Check sheet for the drawn part. Datum: minimum x, y, z corner. Units: mm. A direction names the side the tool comes from. Round coordinates to 2 decimals unless told otherwise and drop trailing zeros. Loops run counter-clockwise (first coordinate to the right, second up) from the corner with the lowest first, then second, coordinate; pieces in that order, holes last. Notation, with made-up numbers: (62.25, 68.5) - (83.25, 68.5) arc R22 cw to (83.25, 104.5) - close; hole circle Ø2 at (62.25, -40). An arc over 180 degrees is marked (long way). Use CSV: the item, a comma, the result in double quotes.
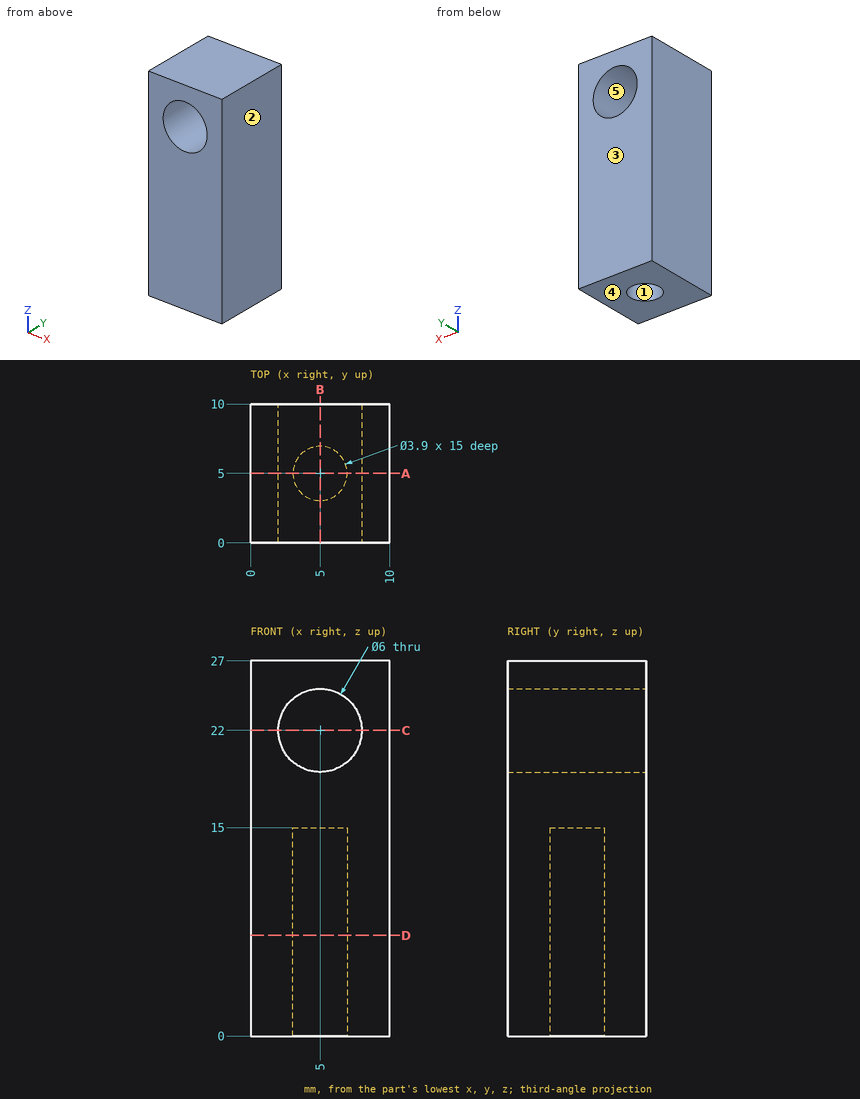
1) Gauge pin test, flat ends, axial feed: pin 1 Ø3 at (x, z) = (4, 22.5) entering from -Y; pin 2 Ø3.5 at (x, y) = (5, 5) entering from -Z. Record the tip position at first contact, or that the pin passes through.
Returned:
pin 1,"passes through"
pin 2,"stops at z = 15"
2) Access from +Z, -Z, +X, -X, +Y, -Y to the whole of each face (thin tool, end or side, straight path). Record for the marked faces 1 and 2.
Returned:
face 1,"-Z"
face 2,"+Z, -Z, +X, +Y, -Y"
3) Cross-section at C-C, the plane z = 22. Record the cut outline in (x, y), then the cut area to 3 significant figures.
Returned:
outline,"(0, 0) - (2, 0) - (2, 10) - (0, 10) - close; (8, 0) - (10, 0) - (10, 10) - (8, 10) - close"
area,"40.0 mm²"
4) Cross-section at B-B, the plane x = 5. Record the cut outline in (y, z).
Returned:
outline,"(0, 0) - (3.05, 0) - (3.05, 15) - (6.95, 15) - (6.95, 0) - (10, 0) - (10, 19) - (0, 19) - close; (0, 25) - (10, 25) - (10, 27) - (0, 27) - close"
5) Thickness scan on probe 1 along Y at (x, z) = (5, 10); probe 2 along Z at (x, y) = (5, 3.5). Record the ranges inside material, lowest first. Write a range as [from, to].
Returned:
probe 1,"y = [0, 3.05], [6.95, 10]"
probe 2,"z = [15, 19], [25, 27]"
6) Cross-section at A-A, the plane y = 5. Record the cut outline in (x, z), then the cut area to 3 significant figures.
Returned:
outline,"(0, 0) - (3.05, 0) - (3.05, 15) - (6.95, 15) - (6.95, 0) - (10, 0) - (10, 27) - (0, 27) - close; hole circle Ø6 at (5, 22)"
area,"183 mm²"
7) Mould release check, pull along Z, two halves, no side actions. Record for the marked faces 3, 4 and 5: +Z half, -Z half, draft (parallel to the pull), parting line (faces both ways), or undercut.
Returned:
face 3,"draft"
face 4,"-Z half"
face 5,"undercut"
8) Cross-section at D-D, the plane z = 7.25. Record the cut outline in (x, y).
Returned:
outline,"(0, 0) - (10, 0) - (10, 10) - (0, 10) - close; hole circle Ø3.9 at (5, 5)"
